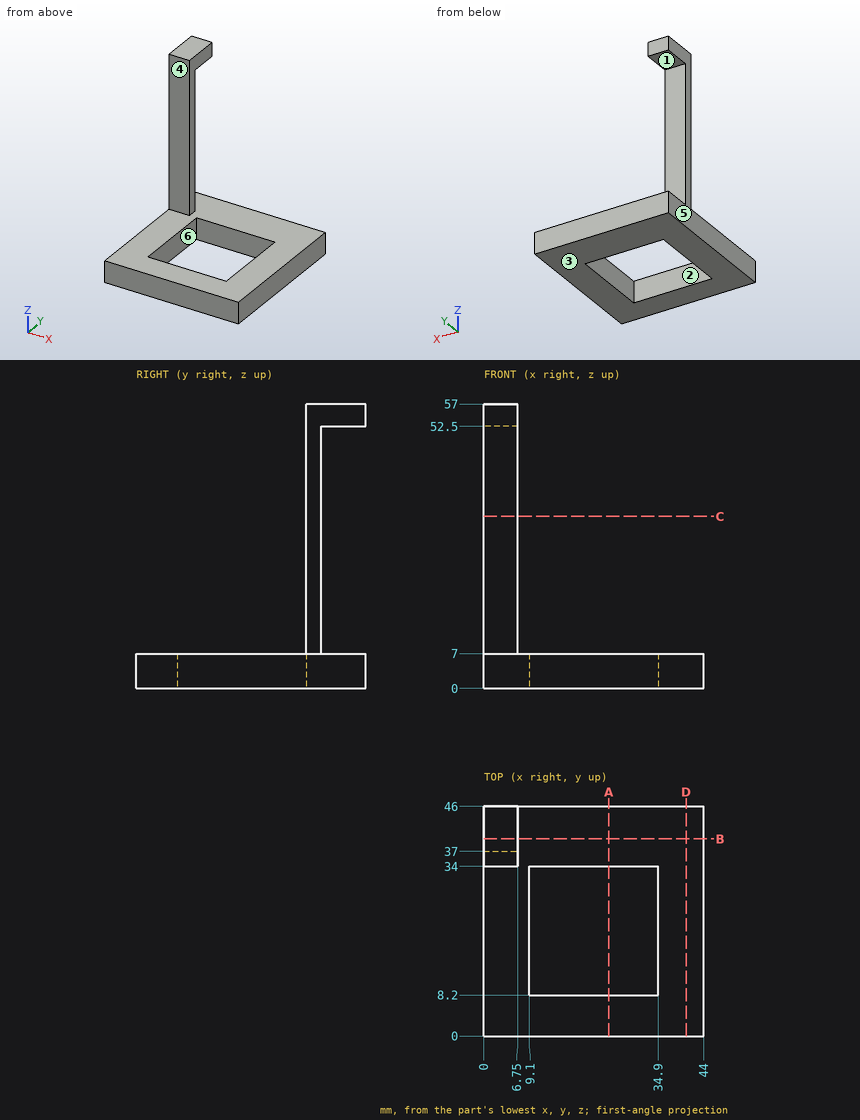
Input: dimensioned drawing with shaded views. Units: mm. Origin: part minimum x, y, z. A direction names the side the tool comes from. Round coordinates to 2 decimals unless told otherwise and drop trailing zeros. Order: outer loops, then holes, each group sorted by start corner. A loop starts at its lowest first (then second) coordinate and runs counter-clockwise, first axis right, second up.
Q1. Pin query (flat end, axial travel): pin 1 (3 mm diameter, centred on y = 40, z = 8, fed in from +X); pin 2 (3.5 mm diameter, centred on y = 39, z = 25, fed in from +X); pin 3 (2 mm diameter, centred on x = 5, z = 39, fed in from +Y); pin 4 (5.5 mm diameter, centred on x = 3.5, z = 20.5, fed in from -Y). Return the tip coordinate at first contact, or that it passes through.
Result sheet:
pin 1: stops at x = 44
pin 2: passes through
pin 3: stops at y = 37
pin 4: stops at y = 34
Q2. Access query for the marked faces 1, 2 and 3. Directions: +Z, -Z, +X, -X, +Y, -Y. A direction counts if a zero-diameter tool reaches every point of the face in a straight line with its end or side. Return the directions, or none.
Result sheet:
face 1: +X, -X, +Y
face 2: +Z, -Z
face 3: -Z, +X, -X, +Y, -Y
Q3. Material intervals for probe 1 along Y at (x, z) = (23, 6.5); probe 2 along Z at (x, y) = (29, 42.5); probe 3 along X at (y, z) = (35, 54), sorted ascending.
Result sheet:
probe 1: y = 0 to 8.2, 34 to 46
probe 2: z = 0 to 7
probe 3: x = 0 to 6.75
Q4. Section D-D, the plane x = 40.5. Output: boundary loops of the cut face in (y, z).
Result sheet:
outline: (0, 0) - (46, 0) - (46, 7) - (0, 7) - close
Q5. Section B-B, the plane y = 39.5. Output: boundary loops of the cut face in (x, z), and give its area (3 significant figures).
Result sheet:
outline: (0, 0) - (44, 0) - (44, 7) - (0, 7) - close; (0, 52.5) - (6.75, 52.5) - (6.75, 57) - (0, 57) - close
area: 338 mm2
Q6. Mould query, pull axis Y, two halves, no side actions, for the marked faces 4, 5 and 6. Classes: released by +Y, released by -Y, zero draft, split by the parting line, or undercut.
Result sheet:
face 4: released by -Y
face 5: zero draft
face 6: undercut
Q7. Section C-C, the plane z = 34.5. Output: boundary loops of the cut face in (x, y).
Result sheet:
outline: (0, 34) - (6.75, 34) - (6.75, 37) - (0, 37) - close
Q8. Section A-A, the plane x = 25. Output: boundary loops of the cut face in (y, z), and give its area (3 significant figures).
Result sheet:
outline: (0, 0) - (8.2, 0) - (8.2, 7) - (0, 7) - close; (34, 0) - (46, 0) - (46, 7) - (34, 7) - close
area: 141 mm2
